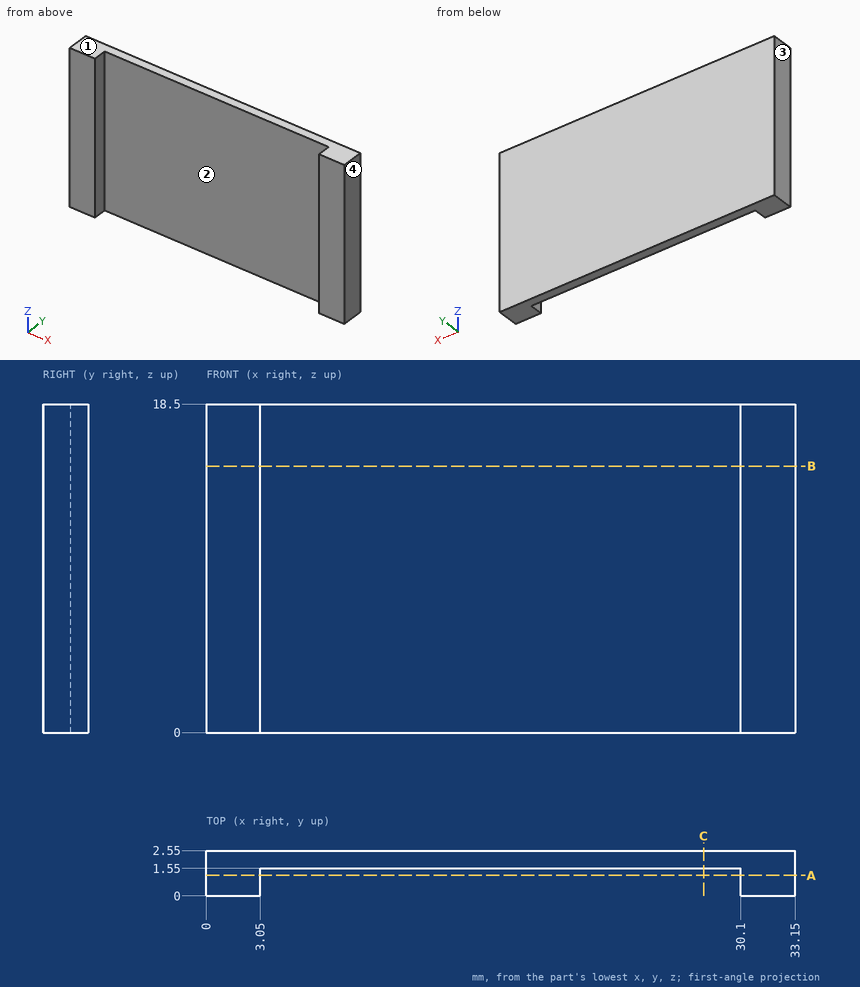
Source: three-view drawing plus pictorial views. Frame: mm from the lowest corner of the part. Round coordinates to 2 decimals unless told otherwise and drop trailing zeros. Order: outer loops, then holes, each group sorted by start corner. A loop starts at its lowest first (then second) coordinate and runs counter-clockwise, first axis right, second up. Notation, with made-up numbers: (29.5, -21) -> (38.5, -21) arc R11 cw to (38.5, -12) -> close; hole circle Ø5 at (19.5, 38.5). An arc over 180 degrees is marked (long way). Use one line per item in the form item = value.
(1) Ray query, probe 1 along X at (y, z) = (1.25, 12.75); probe 2 along Y at (x, z) = (16, 2.25). Return the intervals inside material, ascending. Write a range as [from, to].
Results list:
probe_1 = [0, 3.05], [30.1, 33.15]
probe_2 = [1.55, 2.55]
(2) Section B-B on z = 15. Return loops of the section in (x, y), and give its area (3 significant figures).
Results list:
outline = (0, 0) -> (3.05, 0) -> (3.05, 1.55) -> (30.1, 1.55) -> (30.1, 0) -> (33.15, 0) -> (33.15, 2.55) -> (0, 2.55) -> close
area = 42.6 mm^2
(3) First-contact query: pin 1 Ø0.8 at (y, z) = (1, 12.5) entering from -X. Flat tip, straight axial feed; report the tip coordinate or a pass-through.
Results list:
pin_1 = 0
(4) Draft query along X for the marked faces 1, 2, 3 and 4. Return one class per face: pulls with the +X half, pulls with the -X half, needs draft (parallel to the pull), parting line crosses it, or undercut.
Results list:
face_1 = needs draft
face_2 = undercut
face_3 = pulls with the -X half
face_4 = pulls with the +X half
(5) Section A-A on y = 1.15. Return loops of the section in (x, z), and give its area (3 significant figures).
Results list:
outline = (0, 0) -> (3.05, 0) -> (3.05, 18.5) -> (0, 18.5) -> close; (30.1, 0) -> (33.15, 0) -> (33.15, 18.5) -> (30.1, 18.5) -> close
area = 113 mm^2
(6) Section C-C on x = 28. Return loops of the section in (y, z), and give its area (3 significant figures).
Results list:
outline = (1.55, 0) -> (2.55, 0) -> (2.55, 18.5) -> (1.55, 18.5) -> close
area = 18.5 mm^2
